Source: CAD feature listing. Evaluate the final solid. Frame: model axes, mm. A direction names the side the tool comes from. Round coordinates to 2 decimals unless told otherwise and drop trailing zeros. Order: outer loops, then holes, each group sorted by start corner. A loop starts at its lowest first (then second) coordinate and runs counter-clockwise, first axis right, second up. Notation, with made-up numbers: M 22,-31 L 61,-31 A16 ccw 61,-24 Z; hole C 87,11 d2. An arc over 180 degrees is marked long. Answer as CSV lines item,"result". Start each with the question number.
Item 1: First-contact query: P1, Ø6, axis at x = -11, z = -12, coming from the +Y side; P2, Ø1.5, axis at y = 14, z = 5.5, coming from the +X side; P3, Ø8, axis at y = 2.5, z = 9, coming from the -X side. Flat tips, straight axial feed; report the tip coordinate or a pass-through.
Item 2: Section query C-C on y = 5.25. Return the cut outline in (x, z).
Item 3: Pull-direction query (X, two-part tool) for faces 4 (the face through (-9.76, 13.45, -2.17)), 5 (the face through (-1.3, 15.5, 6.5)), 6 (the face through (-2, 17, 2)); classes: +X half, -X half, draft (parallel to the pull), parting line (faces both ways), or undercut.
Item 4: Section query D-D on y = 14.05. Return the cut outline in (x, z), plus the area to 3 significant figures.
Item 5: Set-up query: faces 1 (the face through (0.325, 15.514, 8.226)), 2 (the face through (0.1, 8.4, -2.6)), 3 (the face through (2.8, 14, 5)). Return all of +Z, -Z, +X, -X, +Y, -Y with unobstructed straight access to the full face (end or side cutting, diameter ignored); none if empty.
Item 6: Section query A-A on x = 0. Return the cut outline in (y, z).
Item 7: Line query: line 1 (X direction, y = 10.5, z = 0); line 2 (X direction, y = 8.5, z = 0); line 3 (Z direction, x = 0.5, y = 16.25). Output: solid intervals per line, ascending. Write a range as [from, to].
Item 8: Section query B-B on z = 0. Return the cut outline in (x, y), plus the area to 3 significant figures.
from build123d import *

# Parameters (mm, degrees)
PULLYBODY_R         = 24
PULLYBODY_R_2       = 2.6
BOSS_EXTRUDE1_DEPTH = 10
SKETCH2_R           = 10
SKETCH2_R_2         = 2.6
BOSS_EXTRUDE2_DEPTH = 7
SKETCH3_W           = 5.6
SKETCH3_H           = 2.5
CUT_EXTRUDE1_DEPTH  = 5.6
SKETCH4_R           = 1.5
CUT_EXTRUDE2_DEPTH  = 38.960505792


with BuildPart() as part:
    # PullyBody → Boss-Extrude1 (new body)
    with BuildSketch(Plane(origin=(0, 0, 0), x_dir=(1, 0, 0), z_dir=(0, 1, 0))):
        with Locations(Location((0, 0, 0), (0, 0, 270))):
            Circle(PULLYBODY_R)
        with Locations(Location((0, 0, 0), (0, 0, 270))):
            Circle(PULLYBODY_R_2, mode=Mode.SUBTRACT)
    extrude(amount=BOSS_EXTRUDE1_DEPTH)

    # Sketch2 → Boss-Extrude2 (add)
    with BuildSketch(Plane(origin=(0, 10, 0), x_dir=(1, 0, 0), z_dir=(0, 1, 0))):
        with Locations(Location((0, 0, 0), (0, 0, 270))):
            Circle(SKETCH2_R)
        with Locations(Location((0, 0, 0), (0, 0, 270))):
            Circle(SKETCH2_R_2, mode=Mode.SUBTRACT)
    extrude(amount=BOSS_EXTRUDE2_DEPTH)

    # Sketch3 → Cut-Extrude1 (cut)
    with BuildSketch(Plane(origin=(0, 17, 0), x_dir=(1, 0, 0), z_dir=(0, 1, 0))):
        with Locations((0, -5.25)):
            Rectangle(SKETCH3_W, SKETCH3_H)
    extrude(amount=-CUT_EXTRUDE1_DEPTH, mode=Mode.SUBTRACT)

    # Sketch4 → Cut-Extrude2 (cut, through all)
    with BuildSketch(Plane.XY):
        with Locations(Location((0, 14.05, 0), (0, 0, 180))):
            Circle(SKETCH4_R)
    extrude(amount=CUT_EXTRUDE2_DEPTH, mode=Mode.SUBTRACT)


solid = part.part
Results:
1,P1,"y = 10"
1,P2,"x = 8.8"
1,P3,"x = -23.47"
2,outline,"C 0,0 d48; hole C 0,0 d5.2"
3,face 4,"parting line"
3,face 5,"undercut"
3,face 6,"draft"
4,outline,"M -2.8,4 L -2.8,6.5 L -1.5,6.5 L -1.5,9.89 A10 ccw long 1.5,9.89 L 1.5,6.5 L 2.8,6.5 L 2.8,4 L 1.5,4 L 1.5,2.12 A2.6 cw long -1.5,2.12 L -1.5,4 Z"
4,area,"264 mm^2"
5,face 1,"+Z"
5,face 2,"+Y, -Y"
5,face 3,"+Y"
6,outline,"M 0,-24 L 10,-24 L 10,-10 L 17,-10 L 17,-2.6 L 0,-2.6 Z; M 0,2.6 L 12.55,2.6 L 12.55,4 L 11.4,4 L 11.4,6.5 L 12.55,6.5 L 12.55,10 L 10,10 L 10,24 L 0,24 Z; M 15.55,2.6 L 17,2.6 L 17,4 L 15.55,4 Z; M 15.55,6.5 L 17,6.5 L 17,10 L 15.55,10 Z"
7,line 1,"[-10, -2.6], [2.6, 10]"
7,line 2,"[-24, -2.6], [2.6, 24]"
7,line 3,"[-9.99, -2.55], [2.55, 4], [6.5, 9.99]"
8,outline,"M -24,0 L -2.6,0 L -2.6,17 L -10,17 L -10,10 L -24,10 Z; M 2.6,0 L 24,0 L 24,10 L 10,10 L 10,17 L 2.6,17 Z"
8,area,"532 mm^2"
